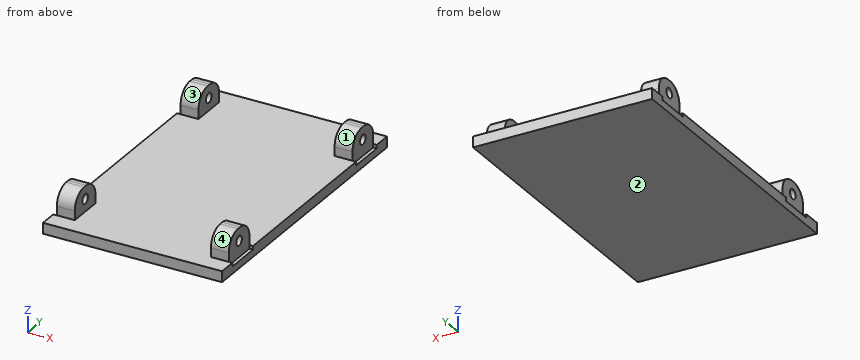
from build123d import *

# Parameters (mm, degrees)
F0_W      = 50
F0_H      = 80
F1_DEPTH  = 3
F2_W      = 6
F2_H      = 10
F3_DEPTH  = 7
F4_R      = 1.35
F5_DEPTH  = 50.001
F6_R      = 4.5
F7_R      = 1.35
F8_DEPTH  = 1
F9_R      = 1.35
F10_DEPTH = 1
F11_W     = 1
F11_H     = 10
F12_DEPTH = 1


with BuildPart() as f1:
    # F0 (on Top) → F1 (new body)
    with BuildSketch(Plane.XY):
        Rectangle(F0_W, F0_H)
    extrude(amount=F1_DEPTH)

    # F2 (on face) → F3 (join)
    with BuildSketch(Plane.XY.offset(3)):
        with Locations((-22, 30)):
            Rectangle(F2_W, F2_H)
        with Locations((22, 30)):
            Rectangle(F2_W, F2_H)
        with Locations((-22, -30)):
            Rectangle(F2_W, F2_H)
        with Locations((22, -30)):
            Rectangle(F2_W, F2_H)
    extrude(amount=F3_DEPTH)

    # F4 (on face) → F5 (cut, through all)
    with BuildSketch(Plane.YZ.offset(25)):
        with Locations((-30, 6.5)):
            Circle(F4_R)
        with Locations((30, 6.5)):
            Circle(F4_R)
    extrude(amount=-F5_DEPTH, mode=Mode.SUBTRACT)

    # F6
    f6_edges = [f1.edges().sort_by_distance(p)[0] for p in [
        (22, -35, 10),
        (22, -25, 10),
        (-22, -35, 10),
        (-22, -25, 10),
        (-22, 25, 10),
        (-22, 35, 10),
        (22, 25, 10),
        (22, 35, 10),
    ]]
    fillet(f6_edges, radius=F6_R)

    # F7 (on face) → F8 (cut)
    with BuildSketch(Plane.YZ.offset(25)):
        with BuildLine():
            Line((-35, 5.5), (-35, 3))
            Line((-35, 3), (-25, 3))
            Line((-25, 3), (-25, 5.5))
            ThreePointArc((-25, 5.5), (-26.3180194847, 8.6819805153), (-29.5, 10))
            Line((-29.5, 10), (-30.5, 10))
            ThreePointArc((-30.5, 10), (-33.6819805153, 8.6819805153), (-35, 5.5))
        make_face()
        with Locations((-30, 6.5)):
            Circle(F7_R, mode=Mode.SUBTRACT)
        with BuildLine():
            Line((25, 5.5), (25, 3))
            Line((25, 3), (35, 3))
            Line((35, 3), (35, 5.5))
            ThreePointArc((35, 5.5), (33.6819805153, 8.6819805153), (30.5, 10))
            Line((30.5, 10), (29.5, 10))
            ThreePointArc((29.5, 10), (26.3180194847, 8.6819805153), (25, 5.5))
        make_face()
        with Locations((30, 6.5)):
            Circle(F7_R, mode=Mode.SUBTRACT)
    extrude(amount=-F8_DEPTH, mode=Mode.SUBTRACT)

    # F9 (on face) → F10 (cut)
    with BuildSketch(Plane(origin=(-25, 0, 0), x_dir=(0, -1, 0), z_dir=(-1, 0, 0))):
        with BuildLine():
            Line((-35, 5.5), (-35, 3))
            Line((-35, 3), (-25, 3))
            Line((-25, 3), (-25, 5.5))
            ThreePointArc((-25, 5.5), (-26.3180194847, 8.6819805153), (-29.5, 10))
            Line((-29.5, 10), (-30.5, 10))
            ThreePointArc((-30.5, 10), (-33.6819805153, 8.6819805153), (-35, 5.5))
        make_face()
        with Locations((-30, 6.5)):
            Circle(F9_R, mode=Mode.SUBTRACT)
        with BuildLine():
            Line((25, 5.5), (25, 3))
            Line((25, 3), (35, 3))
            Line((35, 3), (35, 5.5))
            ThreePointArc((35, 5.5), (33.6819805153, 8.6819805153), (30.5, 10))
            Line((30.5, 10), (29.5, 10))
            ThreePointArc((29.5, 10), (26.3180194847, 8.6819805153), (25, 5.5))
        make_face()
        with Locations((30, 6.5)):
            Circle(F9_R, mode=Mode.SUBTRACT)
    extrude(amount=-F10_DEPTH, mode=Mode.SUBTRACT)

    # F11 (on face) → F12 (cut)
    with BuildSketch(Plane.XY.offset(3)):
        with Locations((-24.5, 30)):
            Rectangle(F11_W, F11_H)
        with Locations((24.5, 30)):
            Rectangle(F11_W, F11_H)
        with Locations((24.5, -30)):
            Rectangle(F11_W, F11_H)
        with Locations((-24.5, -30)):
            Rectangle(F11_W, F11_H)
    extrude(amount=-F12_DEPTH, mode=Mode.SUBTRACT)


solid = f1.part
Can you work these out from the model? Positions are in its coordinate system, mm. Face numbers are marked on the shaded views. Round coordinates to 2 decimals unless told otherwise and drop trailing zeros. Loops run counter-clockwise (first coordinate to the right, second up) from the corner with the lowest first, then second, coordinate; pieces in that order, holes last. Notation, with made-up numbers: (66.5, 0.5) - (70.5, 0.5) arc R28 ccw to (70.5, 21.5) - close; hole circle Ø6 at (68.25, 41). An arc over 180 degrees is marked (long way). Use CSV: the item, a comma, the result in double quotes. Start each with the question number.
1) If we section it at A-A on z = 4.25: Write out the boundary of the cut face in (x, y).
2) If we section it at B-B on y = 21: Write out the boundary of the cut face in (x, z), plus the area to 3 significant figures.
3) Please list where these lines run through material, in increasing order: probe 1 along Z at (x, y) = (-22.8, -30); probe 2 along X at (y, z) = (27, 5.75); probe 3 along Z at (x, y) = (18, -36). Write a range as [from, to].
4) If we section it at C-C on x = 11: Write out the boundary of the cut face in (y, z).
5) For pin 1 Ø0.8 at (x, z) = (-22, 4.5) entering from +Y; pin 2 Ø3.5 at (y, z) = (31.5, 6) entering from -X; pin 3 Ø2 at (y, z) = (27.5, 7.5) entering from +X; pin 4 Ø8 at (x, y) = (-10, 31.5) entering from -Z, each with a flat end and sliding along its axis, tell me the tip position at first contact or that it passes through.
6) We'd pull the mould along Y, two halves only. Please class the marked faces 1, 2, 3 and 4: released by +Y, released by -Y, zero draft, split by the parting line, or undercut.
Geometry results:
1,outline,"(-24, -35) - (-19, -35) - (-19, -25) - (-24, -25) - close; (-24, 25) - (-19, 25) - (-19, 35) - (-24, 35) - close; (19, -35) - (24, -35) - (24, -25) - (19, -25) - close; (19, 25) - (24, 25) - (24, 35) - (19, 35) - close"
2,outline,"(-25, 0) - (25, 0) - (25, 3) - (-25, 3) - close"
2,area,"150 mm2"
3,probe 1,"z = [0, 5.15], [7.85, 10]"
3,probe 2,"x = [-24, -19], [19, 24]"
3,probe 3,"z = [0, 3]"
4,outline,"(-40, 0) - (40, 0) - (40, 3) - (-40, 3) - close"
5,pin 1,"stops at y = 35"
5,pin 2,"stops at x = -24"
5,pin 3,"stops at x = 24"
5,pin 4,"stops at z = 0"
6,face 1,"undercut"
6,face 2,"zero draft"
6,face 3,"undercut"
6,face 4,"released by -Y"
